from build123d import *

# Parameters (mm, degrees)
F1_DEPTH    = 6
F2_T1_DEPTH = 242.8543856465
F3_W        = 10
F3_H        = 30
F4_DEPTH    = 6
F5_R        = 1.5
F6_DEPTH    = 10


# Not quite as in the source:
# - a fillet or chamfer that OpenCascade refuses, or shapes differently, is made with other operations: its cross-section is extruded or revolved along the edge and cut away or added


with BuildPart() as f1:
    # F0 (on Top) → F1 (new body)
    with BuildSketch(Plane.XY):
        Polygon((14.9102990106, 227.5062542017), (-19.0897009894, 227.5062542017), (-19.0897009894, -42.4937457983), (-9.0897009894, -42.4937457983), (-9.0897009894, 87.5062542017), (-7.0897009894, 87.5062542017), (-7.0897009894, -72.4937457983), (2.9102990106, -72.4937457983), (2.9102990106, 87.5062542017), (4.9102990106, 87.5062542017), (4.9102990106, -42.4937457983), (14.9102990106, -42.4937457983), align=None)
    extrude(amount=F1_DEPTH)

    # F2: fillet of radius 50 on 1 edges, made by hand

    # F2_s2 → F2_t1 (cut)
    with BuildSketch(Plane.XY.offset(-118.4271928233)):
        with BuildLine():
            ThreePointArc((14.9102990106, 227.5062542017), (-9.7098930126, 209.2901365467), (-19.0897009894, 180.1353770724))
            Line((-19.0897009894, 180.1353770724), (-19.0897009894, 227.5062542017))
            Line((-19.0897009894, 227.5062542017), (14.9102990106, 227.5062542017))
        make_face()
    extrude(amount=F2_T1_DEPTH, mode=Mode.SUBTRACT)

    # F3 (on face) → F4 (join)
    with BuildSketch(Plane.XY.offset(6)):
        with Locations((-2.0897009894, -57.4937457983)):
            Rectangle(F3_W, F3_H)
    extrude(amount=F4_DEPTH)

    # F5 (on face) → F6 (cut, through all)
    with BuildSketch(Plane(origin=(-7.0897009894, 0, 0), x_dir=(0, -1, 0), z_dir=(-1, 0, 0))):
        with Locations((59.0019002557, 6)):
            Circle(F5_R)
    extrude(amount=-F6_DEPTH, mode=Mode.SUBTRACT)


solid = f1.part
Here's how the part is built. I have some questions about the finished solid (model axes, mm). A direction names the side the tool comes from. Give positions to 0.01 mm unless a question says otherwise; leave off trailing zeros. Loops run counter-clockwise (first coordinate to the right, second up) from the corner with the lowest first, then second, coordinate; pieces in that order, holes last. Notation, with made-up numbers: (-4.75, 52) -> (3.25, 52) arc R17 ccw to (3.25, 59) -> close; hole circle Ø7 at (1.25, -28). An arc over 180 degrees is marked (long way). One line per item, written item: value.
Q1. Suppose I cut it at D-D on x = -14.5. Please give me the cut outline in (y, z).
Answers follow:
outline: (-42.49, 0) -> (201.06, 0) -> (201.06, 6) -> (-42.49, 6) -> close
Q2. We'd pull the mould along X, two halves only. Please class faces 1 (the face through (-14, -42.494, 3)), 2 (the face through (-9.09, 22, 3)), 3 (the face through (-19.09, 70, 3)): pulls with the +X half, pulls with the -X half, needs draft (parallel to the pull), parting line crosses it, or undercut.
Answers follow:
face 1: needs draft
face 2: undercut
face 3: pulls with the -X half
Q3. I'm going to push flat-ended pins straight in: pin 1 Ø6 at (x, y) = (-15.5, 94.5) entering from -Z; pin 2 Ø3 at (x, z) = (-4, 10) entering from +Y; pin 3 Ø1.8 at (y, z) = (-59, 6) entering from +X; pin 4 Ø1.8 at (x, z) = (-13.5, 4.5) entering from -Y. Where does each tip first touch, or does it pass through?
Answers follow:
pin 1: z = 0
pin 2: y = -42.49
pin 3: through
pin 4: y = -42.49
Q4. Suppose I cut it at B-B on z = 2. Please give me the cut outline in (x, y).
Answers follow:
outline: (-19.09, -42.49) -> (-9.09, -42.49) -> (-9.09, 87.51) -> (-7.09, 87.51) -> (-7.09, -72.49) -> (2.91, -72.49) -> (2.91, 87.51) -> (4.91, 87.51) -> (4.91, -42.49) -> (14.91, -42.49) -> (14.91, 227.51) arc R50 ccw to (-19.09, 180.14) -> close
Q5. Suppose I cut it at A-A on y = 4.5. Please give me the cut outline in (x, z).
Answers follow:
outline: (-19.09, 0) -> (-9.09, 0) -> (-9.09, 6) -> (-19.09, 6) -> close; (-7.09, 0) -> (2.91, 0) -> (2.91, 6) -> (-7.09, 6) -> close; (4.91, 0) -> (14.91, 0) -> (14.91, 6) -> (4.91, 6) -> close
Q6. Suppose I cut it at C-C on y = 118. Please give me the cut outline in (x, z).
Answers follow:
outline: (-19.09, 0) -> (14.91, 0) -> (14.91, 6) -> (-19.09, 6) -> close
Q7. If I drill on line 1 along X through (y, z) = (52.5, 3); line 2 along Z through (x, y) = (-9, 206); line 3 along X through (y, z) = (-53.5, 0.75), over which ranges is the centre line in solid material (lowest first)?
Answers follow:
line 1: -19.09 to -9.09, -7.09 to 2.91, 4.91 to 14.91
line 2: 0 to 6
line 3: -7.09 to 2.91
Q8. On a 3-axis mill with a long thin cutter (end or side, diameter ignored), from which of +Z, -Z, +X, -X, +Y, -Y can I reach the whole of each face in a straight line? I mean faces 4 (the face through (-2, 94, 6)), 5 (the face through (-2, -57, 12)), 6 (the face through (10, -42.494, 3)), 7 (the face through (14.91, 91, 3)), 8 (the face through (-7.09, -11, 5)). Say none if no direction works.
Answers follow:
face 4: +Z, +X, -X, +Y
face 5: +Z, +X, -X, +Y, -Y
face 6: +Z, -Z, +X, -Y
face 7: +Z, -Z, +X, +Y, -Y
face 8: +Z, -Z, -Y
